from build123d import *

# Parameters (mm, degrees)
EXTRUDE_1_DEPTH          = 27.5
HOLE_WIZARD_M10_1_D      = 8.5
SKETCH_6_R               = 3.4
CUT_EXTRUDE_1_DEPTH      = 10
SKETCH_9_R               = 5
CUT_EXTRUDE_2_DEPTH      = 136
CUT_EXTRUDE_3_DEPTH      = 1
CUT_EXTRUDE_3_DEPTH_BACK = 109
SKETCH_14_R              = 5.5
CUT_EXTRUDE_5_DEPTH      = 108


with BuildPart() as part:
    # 草圖1 → 填料-伸長1 (new body, symmetric)
    with BuildSketch(Plane.XY):
        with BuildLine():
            Line((0, -54), (-45, -54))
            ThreePointArc((-45, -54), (-48.535533906, -52.535533906), (-50, -49))
            Line((-50, -49), (-50, 49))
            ThreePointArc((-50, 49), (-48.535533906, 52.535533906), (-45, 54))
            Line((-45, 54), (0, 54))
            Line((0, 54), (0, 48))
            Line((0, 48), (-44, 48))
            Line((-44, 48), (-44, -48))
            Line((-44, -48), (0, -48))
            Line((0, -48), (0, -54))
        make_face()
    extrude(amount=EXTRUDE_1_DEPTH, both=True)

    # M10 螺紋孔1 (through all)
    with Locations(Plane(origin=(0, 54, 0), x_dir=(1, 0, 0), z_dir=(0, 1, 0))):
        with Locations((-21, 0)):
            Hole(HOLE_WIZARD_M10_1_D / 2)

    # 草圖6 → 除料-伸長1 (cut)
    with BuildSketch(Plane.ZY.offset(50)):
        with Locations((12.75, 12.75)):
            Circle(SKETCH_6_R)
        with Locations((-12.75, 12.75)):
            Circle(SKETCH_6_R)
        with Locations((-12.75, -12.75)):
            Circle(SKETCH_6_R)
        with Locations((12.75, -12.75)):
            Circle(SKETCH_6_R)
    extrude(amount=-CUT_EXTRUDE_1_DEPTH, mode=Mode.SUBTRACT)

    # 草圖9 → 除料-伸長2 (cut)
    with BuildSketch(Plane(origin=(0, 54, 0), x_dir=(1, 0, 0), z_dir=(0, 1, 0))):
        with Locations((-21, 0)):
            Circle(SKETCH_9_R)
    extrude(amount=-CUT_EXTRUDE_2_DEPTH, mode=Mode.SUBTRACT)

    # 草圖10 → 除料-伸長3 (cut, two sides)
    with BuildSketch(Plane(origin=(0, 54, 0), x_dir=(1, 0, 0), z_dir=(0, 1, 0))) as cut_extrude_3_sk:
        with BuildLine():
            Line((-180.04752128, 68.815685703), (-40, 27.5))
            Line((-40, 27.5), (-15.057931362, 20.141792877))
            ThreePointArc((-15.057931362, 20.141792877), (0, 0), (-15.057931362, -20.141792877))
            Line((-15.057931362, -20.141792877), (-40, -27.5))
            Line((-40, -27.5), (-180.04752128, -68.815685703))
            Line((-180.04752128, -68.815685703), (111.981888895, -68.815685703))
            Line((111.981888895, -68.815685703), (111.981888895, 68.815685703))
            Line((111.981888895, 68.815685703), (-180.04752128, 68.815685703))
        make_face()
    extrude(amount=CUT_EXTRUDE_3_DEPTH, mode=Mode.SUBTRACT)
    extrude(cut_extrude_3_sk.sketch, amount=-CUT_EXTRUDE_3_DEPTH_BACK, mode=Mode.SUBTRACT)

    # 草圖14 → 除料-伸長5 (cut)
    with BuildSketch(Plane(origin=(0, 54, 0), x_dir=(1, 0, 0), z_dir=(0, 1, 0))):
        with Locations((-21, 0)):
            Circle(SKETCH_14_R)
    extrude(amount=-CUT_EXTRUDE_5_DEPTH, mode=Mode.SUBTRACT)


solid = part.part
Can you work these out from the model? Positions are in its coordinate system, mm. A direction names the side the tool comes from. Give positions to 0.01 mm unless a question says otherwise; leave off trailing zeros. Loops run counter-clockwise (first coordinate to the right, second up) from the corner with the lowest first, then second, coordinate; pieces in that order, holes last. Notation, with made-up numbers: (15.5, 68.25) - (70.5, 68.25) arc R27 cw to (70.5, 106.25) - close; hole circle Ø11 at (61, 76.25). An arc over 180 degrees is marked (long way). Answer as a JSON object with one key per item and string values.
Q1. If we mould it in two halves opening along Z, with no side actions, what happens to faces 1 (the cylindrical face through (-47.04, -16.07, 12.01)), 2 (the flat face through (-27.7, 51.04, -23.87)), 3 (the flat face through (-47, 1, 27.5))? For each: pulls with the +Z half, pulls with the -Z half, needs draft (parallel to the pull), parting line crosses it, or undercut.
Geometry says:
{"face 1": "undercut", "face 2": "pulls with the -Z half", "face 3": "pulls with the +Z half"}
Q2. Imagine slicing it at D-D on x = -42. Write out the boundary of the cut face in (y, z).
Geometry says:
{"outline": "(-54, -27.5) - (-48, -27.5) - (-48, 27.5) - (-54, 27.5) - close; (48, -27.5) - (54, -27.5) - (54, 27.5) - (48, 27.5) - close"}
Q3. Will these pins go through, and if not, where does the flat tip stop? P1, Ø4, axis at y = 12.75, z = -12.75, coming from the -X side; P2, Ø12, axis at y = -37, z = -3.5, coming from the +X side.
Geometry says:
{"P1": "through", "P2": "x = -44"}
Q4. Imagine slicing it at A-A on z = 0. Write out the boundary of the cut face in (x, y).
Geometry says:
{"outline": "(-50, -49) arc R5 ccw to (-45, -54) - (-26.5, -54) - (-26.5, -48) - (-44, -48) - (-44, 48) - (-26.5, 48) - (-26.5, 54) - (-45, 54) arc R5 ccw to (-50, 49) - close; (-15.5, -54) - (0, -54) - (0, -48) - (-15.5, -48) - close; (-15.5, 48) - (0, 48) - (0, 54) - (-15.5, 54) - close"}
Q5. If I drill on L1, parallel to Y at x = -47.3, z = 12.75; L2, parallel to Y at x = -48.65, z = 12.75; L3, parallel to Y at x = -10.5, z = -12.5, over which ranges is the centre line in solid material (lowest first)?
Geometry says:
{"L1": "-53.44 to -16.15, -9.35 to 9.35, 16.15 to 53.44", "L2": "-52.42 to -16.15, -9.35 to 9.35, 16.15 to 52.42", "L3": "-54 to -48, 48 to 54"}
Q6. Imagine slicing it at C-C on x = -22. Write out the boundary of the cut face in (y, z), plus the area to 3 significant figures.
Geometry says:
{"outline": "(-54, -22.19) - (-48, -22.19) - (-48, -5.41) - (-54, -5.41) - close; (-54, 5.41) - (-48, 5.41) - (-48, 22.19) - (-54, 22.19) - close; (48, -22.19) - (54, -22.19) - (54, -5.41) - (48, -5.41) - close; (48, 5.41) - (54, 5.41) - (54, 22.19) - (48, 22.19) - close", "area": "403 mm²"}
Q7. Imagine slicing it at B-B on y = -12.75. Write out the boundary of the cut face in (x, z), plus the area to 3 significant figures.
Geometry says:
{"outline": "(-50, -27.5) - (-44, -27.5) - (-44, -16.15) - (-50, -16.15) - close; (-50, -9.35) - (-44, -9.35) - (-44, 9.35) - (-50, 9.35) - close; (-50, 16.15) - (-44, 16.15) - (-44, 27.5) - (-50, 27.5) - close", "area": "248 mm²"}
Q8. Which directions (+Z, -Z, +X, -X, +Y, -Y) give clear straight access to the entire face, cutting with the end or side of a thin tool? Please do faces 4 (the flat face through (-44, 1, 0)), 5 (the flat face through (-28, 54, 0)).
Geometry says:
{"face 4": "+Z, -Z, +X", "face 5": "+Z, -Z, +X, -X, +Y"}
